```python
from build123d import *

# Parameters (mm, degrees)
EXTRUDE_1_DEPTH     = 142
FILLET_1_R          = 5
SKETCH_2_R          = 4.4
CUT_EXTRUDE_1_DEPTH = 10


with BuildPart() as part:
    # Эскиз1 → Бобышка-Вытянуть1 (new, symmetric)
    with BuildSketch(Plane.XY):
        Polygon((0, 0), (50, 0), (50, -5), (5, -5), (5, -50), (0, -50), align=None)
    extrude(amount=EXTRUDE_1_DEPTH, both=True)

    # Скругление1
    fillet_1_edges = [part.edges().sort_by_distance(p)[0] for p in [
        (5, -5, 0),
    ]]
    fillet(fillet_1_edges, radius=FILLET_1_R)

    # Эскиз2 → Вырез-Вытянуть1 (cut)
    with BuildSketch(Plane(origin=(0, 0, 0), x_dir=(1, 0, 0), z_dir=(0, 1, 0))):
        with Locations(Location((27, 72, 0), (0, 0, 270))):
            Circle(SKETCH_2_R)
    cut_extrude_1 = extrude(amount=-CUT_EXTRUDE_1_DEPTH, mode=Mode.SUBTRACT)

    # Зеркальное отражение1: Вырез-Вытянуть1 across plane
    add(cut_extrude_1.mirror(Plane.XY), mode=Mode.SUBTRACT)


solid = part.part
```
Geometry: final body of the model. Coordinates: model frame, mm. A direction names the side the tool comes from. Give positions to 0.01 mm unless a question says otherwise; leave off trailing zeros. Loops run counter-clockwise (first coordinate to the right, second up) from the corner with the lowest first, then second, coordinate; pieces in that order, holes last. Notation, with made-up numbers: (-38, 37) - (-26, 37) arc R20 cw to (-26, 53) - close; hole circle Ø11 at (71, 62.5). An arc over 180 degrees is marked (long way). Answer as CSV lines item,"result". Start each with the question number.
(1) Reachability of faces 1 (the face through (3, -50, 2)), 2 (the face through (5, -30, 2)) from +Z, -Z, +X, -X, +Y, -Y: full face, straight path, thin tool, end or side. Return the list, or none.
(2) Section query C-C (y = -33). Output: boundary loops of the cut face in (x, z), and give its area (3 significant figures).
(3) Section query D-D (x = 42.5). Output: boundary loops of the cut face in (y, z).
(4) Mould query, pull axis Z, two halves, no side actions, for faces 3 (the face through (27.193, -2.465, 76.396)), 4 (the face through (15.9, -4.5, -142)), 5 (the face through (30, -5, 2)). Classes: +Z half, -Z half, draft (parallel to the pull), parting line (faces both ways), or undercut.
(5) Section query A-A (x = 27). Output: boundary loops of the cut face in (y, z), and give its area (3 significant figures).
(6) Section query B-B (z = -72). Output: boundary loops of the cut face in (x, y).
(7) Pin query (flat end, axial travel): P1, Ø4, axis at x = 39, z = 15.5, coming from the -Y side; P2, Ø4, axis at y = -25.5, z = 107, coming from the +X side; P3, Ø8, axis at x = 27, z = -72, coming from the +Y side. Return the tip coordinate at first contact, or that it passes through.
(8) Ray query, line 1 along X through (y, z) = (-2.65, -72); line 2 along Y through (x, z) = (26.5, -3); line 3 along X through (y, z) = (-33.5, -115.5). Return the intervals inside material, ascending. Write a range as [from, to].
Worked answers:
1,face 1,"+Z, -Z, +X, -X, -Y"
1,face 2,"+Z, -Z, +X, -Y"
2,outline,"(0, -142) - (5, -142) - (5, 142) - (0, 142) - close"
2,area,"1,420 mm^2"
3,outline,"(-5, -142) - (0, -142) - (0, 142) - (-5, 142) - close"
4,face 3,"undercut"
4,face 4,"-Z half"
4,face 5,"draft"
5,outline,"(-5, -142) - (0, -142) - (0, -76.4) - (-5, -76.4) - close; (-5, -67.6) - (0, -67.6) - (0, 67.6) - (-5, 67.6) - close; (-5, 76.4) - (0, 76.4) - (0, 142) - (-5, 142) - close"
5,area,"1,330 mm^2"
6,outline,"(0, -50) - (5, -50) - (5, -10) arc R5 cw to (10, -5) - (22.6, -5) - (22.6, 0) - (0, 0) - close; (31.4, -5) - (50, -5) - (50, 0) - (31.4, 0) - close"
7,P1,"stops at y = -5"
7,P2,"stops at x = 5"
7,P3,"passes through"
8,line 1,"x = [0, 22.6], [31.4, 50]"
8,line 2,"y = [-5, 0]"
8,line 3,"x = [0, 5]"
